The listing builds one solid part. Answer for the finished solid, in the listing's coordinates (mm). A direction names the side the tool comes from. Give positions to 0.01 mm unless a question says otherwise; leave off trailing zeros. Loops run counter-clockwise (first coordinate to the right, second up) from the corner with the lowest first, then second, coordinate; pieces in that order, holes last.
Item 1: Each of these flat-tipped pins is pushed along its axis until it touches: pin 1 Ø7 at (x, z) = (59.5, -12.5) entering from +Y; pin 2 Ø14 at (x, y) = (-43.5, -19.5) entering from +Z; pin 3 Ø5 at (x, y) = (35.5, -30.5) entering from +Z. Where does it stop, or does it pass through?
Item 2: A tool of negligible diameter and unlimited length cuts with its end or side. For faces 4 (the face through (21.486, -30.907, -11.724)), 5 (the face through (-27.771, -31.306, 9.043)), 6 (the face through (55, -23, 0)), 7 (the face through (56, -43.749, -12)), 8 (the face through (57, -18.498, -12)), from which of +Z, -Z, +X, -X, +Y, -Y can it reach the whole face along a straight path? Write none if from no direction.
Item 3: Section C-C, the plane z = 8.5 is taken. Give the vertices of the cut face in (x, y).
Item 4: Consider line 1 along Y through (x, z) = (59, -3); line 2 along X through (y, z) = (-60, -16); line 3 along X through (y, z) = (-27.5, -22.5). Determine where each line is inside the solid, lowest interval first.
Item 5: The mould has two halves that part along Y. Classify faces 1 (the face through (89.85, -31.33, -11.72)), 2 (the face through (56, -24.37, -12)), 3 (the face through (-51.775, -31, -3)): pulls with the +Y half, pulls with the -Y half, needs draft (parallel to the pull), parting line crosses it, or undercut.
Item 6: Section D-D, the plane x = 67 is taken. Give the vertices of the cut face in (y, z), and give its area (3 significant figures).
Item 7: Section A-A, the plane z = -9 is taken. Give the vertices of the cut face in (x, y).
Item 8: Section B-B, the plane y = -8 is taken. Give the vertices of the cut face in (x, z).
from build123d import *

# Parameters (mm, degrees)
F1_DEPTH = 63.5
F3_DEPTH = 25.4


with BuildPart() as f1:
    # F0 (on Front) → F1 (new body)
    with BuildSketch(Plane.XZ):
        with BuildLine():
            Line((-97.852716, 24.277382), (-97.852716, -46.572937))
            Line((-97.852716, -46.572937), (102.807284, -46.572937))
            Line((102.807284, -46.572937), (102.807284, -23.781926))
            Line((102.807284, -23.781926), (5.920396, -23.781926))
            ThreePointArc((5.920396, -23.781926), (1.430268, -21.922054), (-0.429604, -17.431926))
            Line((-0.429604, -17.431926), (-0.429604, 17.836444))
            Line((-0.429604, 17.836444), (-16.779679, 17.836444))
            Line((-16.779679, 17.836444), (-39.075235, 0))
            Line((-39.075235, 0), (-39.075235, -6.440938))
            Line((-39.075235, -6.440938), (-51.775235, -6.440938))
            Line((-51.775235, -6.440938), (-51.775235, 0))
            Line((-51.775235, 0), (-85.466295, 24.277382))
            Line((-85.466295, 24.277382), (-97.852716, 24.277382))
        make_face()
    extrude(amount=F1_DEPTH)

    # F2 (on Top) → F3 (join)
    with BuildSketch(Plane.XY):
        with BuildLine():
            Line((83.36813, -18.497726), (29.049411, -18.497726))
            ThreePointArc((29.049411, -18.497726), (21.484507, -31.123157), (29.049411, -43.748587))
            Line((29.049411, -43.748587), (83.36813, -43.748587))
            ThreePointArc((83.36813, -43.748587), (89.852645, -31.123157), (83.36813, -18.497726))
        make_face()
        with BuildLine():
            ThreePointArc((38.738701, -37.289064), (32.279179, -30.829541), (38.738701, -24.370018))
            Line((38.738701, -24.370018), (74.266076, -24.370018))
            ThreePointArc((74.266076, -24.370018), (80.725599, -30.829541), (74.266076, -37.289064))
            Line((74.266076, -37.289064), (38.738701, -37.289064))
        make_face(mode=Mode.SUBTRACT)
    extrude(amount=-F3_DEPTH)


solid = f1.part
Worked answers:
1. pin 1: stops at y = -18.5
1. pin 2: stops at z = 2.06
1. pin 3: stops at z = -23.78
2. face 4: +Z
2. face 5: +Z, +Y, -Y
2. face 6: +Z, +X, +Y, -Y
2. face 7: +Z, +X, -Y
2. face 8: +Z, +X, +Y
3. outline: (-97.85, -63.5) - (-63.57, -63.5) - (-63.57, 0) - (-97.85, 0) - close; (-28.45, -63.5) - (-0.43, -63.5) - (-0.43, 0) - (-28.45, 0) - close
4. line 1: y = -43.75 to -37.29, -24.37 to -18.5
4. line 2: x = -97.85 to -0.43
4. line 3: x = -97.85 to 2.09, 21.95 to 33.2, 79.8 to 89.42
5. face 1: parting line crosses it
5. face 2: undercut
5. face 3: needs draft
6. outline: (-63.5, -46.57) - (0, -46.57) - (0, -23.78) - (-18.5, -23.78) - (-18.5, 0) - (-24.37, 0) - (-24.37, -23.78) - (-37.29, -23.78) - (-37.29, 0) - (-43.75, 0) - (-43.75, -23.78) - (-63.5, -23.78) - close
6. area: 1,740 mm2
7. outline: (-97.85, -63.5) - (-0.43, -63.5) - (-0.43, 0) - (-97.85, 0) - close; (29.05, -43.75) - (83.37, -43.75) arc R15.53 ccw to (83.37, -18.5) - (29.05, -18.5) arc R14.32 ccw to start; hole (38.74, -37.29) - (74.27, -37.29) arc R6.46 ccw to (74.27, -24.37) - (38.74, -24.37) arc R6.46 ccw to start
8. outline: (-97.85, -46.57) - (102.81, -46.57) - (102.81, -23.78) - (5.92, -23.78) arc R6.35 cw to (-0.43, -17.43) - (-0.43, 17.84) - (-16.78, 17.84) - (-39.08, 0) - (-39.08, -6.44) - (-51.78, -6.44) - (-51.78, 0) - (-85.47, 24.28) - (-97.85, 24.28) - close
